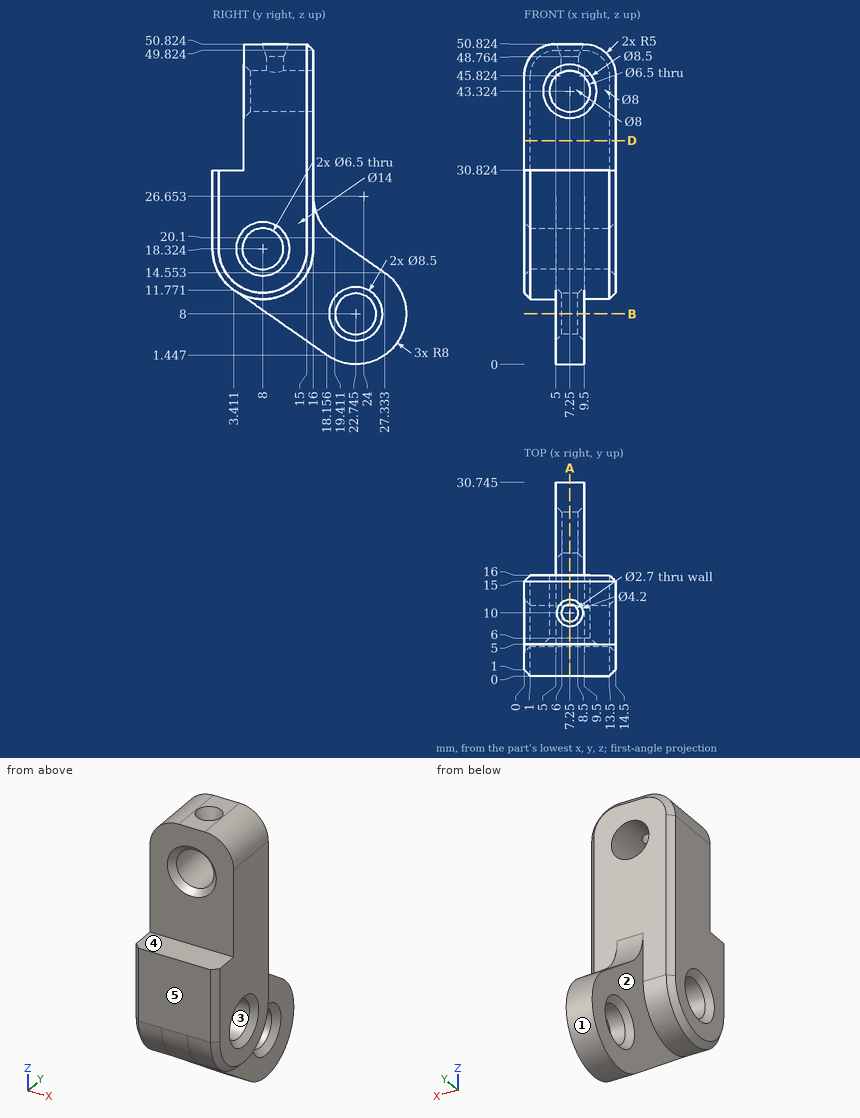
For this review, use the dimensioned drawing (mm, ordinates from the lowest corner) and the shaded views. A direction names the side the tool comes from. Round coordinates to 2 decimals unless told otherwise and drop trailing zeros. Loops run counter-clockwise (first coordinate to the right, second up) from the corner with the lowest first, then second, coordinate; pieces in that order, holes last. Notation, with made-up numbers: M 27,-13 L 78,-13 A11 cw 78,4 Z; hole C 83,77 d1. An arc over 180 degrees is marked long. Answer as a JSON object with one key per item and string values.
(1) Clearance check with flat-ended pins moving along their axes: P1, Ø2, axis at x = 5.5, y = 20, coming from the -Z side; P2, Ø8.5, axis at x = 7.25, z = 43.32, coming from the +Y side; P3, Ø4, axis at x = 10, y = 2, coming from the +Z side. State where each tip first meets the part, or that it passes through.
Resolved:
{"P1": "z = 0.19", "P2": "y = 16", "P3": "z = 30.82"}
(2) Take a section at A-A on x = 7.25. Count the separate pieces of the cut face and the enclosed holes in it, and give its area (3 significant figures).
Resolved:
{"separate pieces": "3", "enclosed holes": "2", "area": "656 mm²"}
(3) Tool access review of the marked faces 4 and 5: name each direction out of +Z, -Z, +X, -X, +Y, -Y from which nothing blocks a thin tool from reaching the whole face with its end or side.
Resolved:
{"face 4": "+Z, +X, -X, -Y", "face 5": "+Z, -Z, +X, -X, -Y"}
(4) Draft analysis for pull direction Y (two halves, no side actions). For the marked faces 1, 2 and 3, state which applies: released by +Y, released by -Y, zero draft, split by the parting line, or undercut.
Resolved:
{"face 1": "split by the parting line", "face 2": "zero draft", "face 3": "undercut"}
(5) Take a section at D-D on z = 35.5. Give the boundary of the cut face in (x, y), and give its area (4 significant figures).
Resolved:
{"outline": "M 0,5 L 14.5,5 L 14.5,15 L 13.5,16 L 1,16 L 0,15 Z", "area": "158.5 mm²"}
(6) Take a section at B-B on z = 8. Give the boundary of the cut face in (x, y) (1 decimal).
Resolved:
{"outline": "M 5,8.8 L 9.5,8.8 L 9.5,18.5 L 8.5,19.5 L 6,19.5 L 5,18.5 Z; M 5,27 L 6,26 L 8.5,26 L 9.5,27 L 9.5,30.7 L 5,30.7 Z"}
(7) To check wall thickness, follow line 1 along Z through (x, y) = (4.25, 7.5) (1 decimal); line 2 along Y through (x, z) = (12.5, 24.5); line 3 along Y through (x, z) = (12.5, 44). State the ranges of each line that lie inside material, in increasing order.
Resolved:
{"line 1": "10.3 to 15.1, 21.5 to 42.1, 44.6 to 50.8", "line 2": "0 to 16", "line 3": "5 to 16"}
